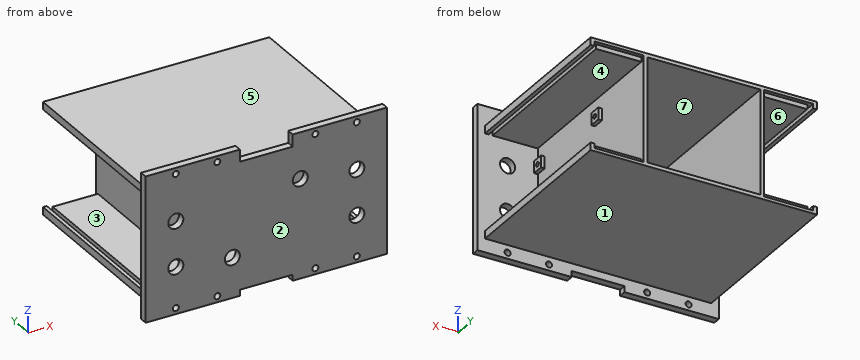
from build123d import *

# Parameters (mm, degrees)
SKETCH1_W               = 203.2
SKETCH1_H               = 203.2
BOSS_EXTRUDE1_DEPTH     = 6.35
SKETCH2_W               = 44.45
SKETCH2_H               = 45.72
SKETCH2_H_2             = 50.8
CUT_EXTRUDE1_DEPTH      = 144.824345992
SKETCH3_R               = 2.54
SKETCH3_W               = 25.4
SKETCH3_H               = 25.4
CUT_EXTRUDE2_DEPTH      = 6.35
MIRROR2_COPY_1_SKETCH_R = 2.54
MIRROR2_COPY_1_SKETCH_W = 25.4
MIRROR2_COPY_1_SKETCH_H = 25.4
MIRROR2_COPY_1_DEPTH    = 6.35
SKETCH4_W               = 101.6
SKETCH4_H               = 93.98
SKETCH4_W_2             = 95.25
SKETCH4_H_2             = 87.63
BOSS_EXTRUDE2_DEPTH     = 152.4
SKETCH5_W               = 10
SKETCH5_H               = 10
SKETCH5_R               = 1.6
BOSS_EXTRUDE3_DEPTH     = 3.175
CUT_EXTRUDE3_REACH      = 246.393
SKETCH8_R               = 1.905
SKETCH9_W               = 6.35
SKETCH9_H               = 152.4
BOSS_EXTRUDE4_DEPTH     = 44.45
SKETCH12_W              = 3.175
SKETCH12_H              = 3.81
CUT_EXTRUDE4_DEPTH      = 152.4
SKETCH13_W              = 38.1
SKETCH13_H              = 3.81
CUT_EXTRUDE5_DEPTH      = 3.175
SKETCH14_W              = 6.35
SKETCH14_H              = 152.4
BOSS_EXTRUDE5_DEPTH     = 44.45
SKETCH15_W              = 3.175
SKETCH15_H              = 3.81
CUT_EXTRUDE6_DEPTH      = 152.4
SKETCH16_W              = 38.1
SKETCH16_H              = 3.81
CUT_EXTRUDE7_DEPTH      = 3.175
CUT_EXTRUDE8_REACH      = 211.454
SKETCH17_R              = 6.35
MIRROR5_OUTLINE_R       = 6.35
MIRROR5_DEPTH           = 6.35
SKETCH18_W              = 79.375
SKETCH18_H              = 40.64
CUT_EXTRUDE9_DEPTH      = 210.453765781


# Read off the part's stored shape, not the designer's step: Mirror5
with BuildPart() as part:
    # Sketch1 → Boss-Extrude1 (new body)
    with BuildSketch(Plane(origin=(0, 0, 0), x_dir=(1, 0, 0), z_dir=(0, 1, 0))):
        Rectangle(SKETCH1_W, SKETCH1_H)
    extrude(amount=BOSS_EXTRUDE1_DEPTH)

    # Sketch2 → Cut-Extrude1 (cut, through all)
    with BuildSketch(Plane(origin=(0, 6.35, 0), x_dir=(1, 0, 0), z_dir=(0, 1, 0))):
        with Locations((0, 78.74)):
            Rectangle(SKETCH2_W, SKETCH2_H)
        with Locations((0, -76.2)):
            Rectangle(SKETCH2_W, SKETCH2_H_2)
    extrude(amount=-CUT_EXTRUDE1_DEPTH, mode=Mode.SUBTRACT)

    # Sketch3 → Cut-Extrude2 (cut)
    with BuildSketch(Plane(origin=(0, 6.35, 0), x_dir=(1, 0, 0), z_dir=(0, 1, 0))):
        with Locations(Location((-96.52, 76.2, 0), (0, 0, 270))):
            Circle(SKETCH3_R)
        with Locations(Location((-76.2, 96.52, 0), (0, 0, 270))):
            Circle(SKETCH3_R)
        with Locations(Location((-76.2, 55.88, 0), (0, 0, 270))):
            Circle(SKETCH3_R)
        with Locations(Location((-41.275, 96.52, 0), (0, 0, 270))):
            Circle(SKETCH3_R)
        with Locations(Location((-41.275, 55.88, 0), (0, 0, 90))):
            Circle(SKETCH3_R)
        with Locations((-41.148, 76.2)):
            Rectangle(SKETCH3_W, SKETCH3_H)
        with Locations((-76.2, 76.2)):
            Rectangle(SKETCH3_W, SKETCH3_H)
    cut_extrude2 = extrude(amount=-CUT_EXTRUDE2_DEPTH, mode=Mode.SUBTRACT)

    # Mirror1: Cut-Extrude2 across plane
    add(cut_extrude2.mirror(Plane(origin=(0, 0, 0), x_dir=(0, 0, 1), z_dir=(1, 0, 0))), mode=Mode.SUBTRACT)

    # Mirror2: Cut-Extrude2 across plane
    add(cut_extrude2.mirror(Plane.XY), mode=Mode.SUBTRACT)

    # Mirror2 copy 1 sketch → Mirror2 copy 1 (cut)
    with BuildSketch(Plane(origin=(0, 6.35, 0), x_dir=(-1, 0, 0), z_dir=(0, 1, 0))):
        with Locations(Location((-96.52, 76.2, 0), (0, 0, 270))):
            Circle(MIRROR2_COPY_1_SKETCH_R)
        with Locations(Location((-76.2, 96.52, 0), (0, 0, 270))):
            Circle(MIRROR2_COPY_1_SKETCH_R)
        with Locations(Location((-76.2, 55.88, 0), (0, 0, 270))):
            Circle(MIRROR2_COPY_1_SKETCH_R)
        with Locations(Location((-41.275, 96.52, 0), (0, 0, 270))):
            Circle(MIRROR2_COPY_1_SKETCH_R)
        with Locations(Location((-41.275, 55.88, 0), (0, 0, 90))):
            Circle(MIRROR2_COPY_1_SKETCH_R)
        with Locations((-41.148, 76.2)):
            Rectangle(MIRROR2_COPY_1_SKETCH_W, MIRROR2_COPY_1_SKETCH_H)
        with Locations((-76.2, 76.2)):
            Rectangle(MIRROR2_COPY_1_SKETCH_W, MIRROR2_COPY_1_SKETCH_H)
    extrude(amount=-MIRROR2_COPY_1_DEPTH, mode=Mode.SUBTRACT)

    # Sketch4 → Boss-Extrude2 (add)
    with BuildSketch(Plane(origin=(0, 6.35, 0), x_dir=(1, 0, 0), z_dir=(0, 1, 0))):
        with Locations((0, 2.54)):
            Rectangle(SKETCH4_W, SKETCH4_H)
        with Locations((0, 2.54)):
            Rectangle(SKETCH4_W_2, SKETCH4_H_2, mode=Mode.SUBTRACT)
    extrude(amount=BOSS_EXTRUDE2_DEPTH)

    # Sketch5 → Boss-Extrude3 (add)
    # profile 1 of 4: a face of its own
    with BuildSketch(Plane(origin=(50.8, 0, 0), x_dir=(0, 0, -1), z_dir=(1, 0, 0))):
        with Locations((-21.59, 93.98)):
            Rectangle(SKETCH5_W, SKETCH5_H)
        with Locations((-21.59, 93.98)):
            Circle(SKETCH5_R, mode=Mode.SUBTRACT)
    # profile 2 of 4: a face of its own
    with BuildSketch(Plane(origin=(50.8, 0, 0), x_dir=(0, 0, -1), z_dir=(1, 0, 0))):
        with Locations((26.67, 92.71)):
            Rectangle(SKETCH5_W, SKETCH5_H)
        with Locations((26.67, 92.71)):
            Circle(SKETCH5_R, mode=Mode.SUBTRACT)
    # profile 3 of 4: a face of its own
    with BuildSketch(Plane(origin=(50.8, 0, 0), x_dir=(0, 0, -1), z_dir=(1, 0, 0))):
        with Locations((-21.59, 11.43)):
            Rectangle(SKETCH5_W, SKETCH5_H)
        with Locations((-21.59, 11.43)):
            Circle(SKETCH5_R, mode=Mode.SUBTRACT)
    # profile 4 of 4: a face of its own
    with BuildSketch(Plane(origin=(50.8, 0, 0), x_dir=(0, 0, -1), z_dir=(1, 0, 0))):
        with Locations((26.67, 17.78)):
            Rectangle(SKETCH5_W, SKETCH5_H)
        with Locations((26.67, 17.78)):
            Circle(SKETCH5_R, mode=Mode.SUBTRACT)
    extrude(amount=BOSS_EXTRUDE3_DEPTH)

    # Sketch8 → Cut-Extrude3 (cut, up to next)
    with BuildSketch(Plane(origin=(53.975, 0, 0), x_dir=(0, 0, -1), z_dir=(1, 0, 0)), mode=Mode.PRIVATE) as cut_extrude3_sk1:
        with Locations((-21.59, 93.98)):
            Circle(SKETCH8_R)
    cut_extrude3_tool1 = extrude(cut_extrude3_sk1.sketch, amount=-CUT_EXTRUDE3_REACH, mode=Mode.PRIVATE) & part.part
    # Sketch8 → Cut-Extrude3 (cut, up to next)
    with BuildSketch(Plane(origin=(53.975, 0, 0), x_dir=(0, 0, -1), z_dir=(1, 0, 0)), mode=Mode.PRIVATE) as cut_extrude3_sk2:
        with Locations((26.67, 92.71)):
            Circle(SKETCH8_R)
    cut_extrude3_tool2 = extrude(cut_extrude3_sk2.sketch, amount=-CUT_EXTRUDE3_REACH, mode=Mode.PRIVATE) & part.part
    # Sketch8 → Cut-Extrude3 (cut, up to next)
    with BuildSketch(Plane(origin=(53.975, 0, 0), x_dir=(0, 0, -1), z_dir=(1, 0, 0)), mode=Mode.PRIVATE) as cut_extrude3_sk3:
        with Locations((-21.59, 11.43)):
            Circle(SKETCH8_R)
    cut_extrude3_tool3 = extrude(cut_extrude3_sk3.sketch, amount=-CUT_EXTRUDE3_REACH, mode=Mode.PRIVATE) & part.part
    # Sketch8 → Cut-Extrude3 (cut, up to next)
    with BuildSketch(Plane(origin=(53.975, 0, 0), x_dir=(0, 0, -1), z_dir=(1, 0, 0)), mode=Mode.PRIVATE) as cut_extrude3_sk4:
        with Locations((26.67, 17.78)):
            Circle(SKETCH8_R)
    cut_extrude3_tool4 = extrude(cut_extrude3_sk4.sketch, amount=-CUT_EXTRUDE3_REACH, mode=Mode.PRIVATE) & part.part
    add(cut_extrude3_tool1.solids().sort_by_distance((53.975, 93.98, 21.59))[0], mode=Mode.SUBTRACT)
    add(cut_extrude3_tool2.solids().sort_by_distance((53.975, 92.71, -26.67))[0], mode=Mode.SUBTRACT)
    add(cut_extrude3_tool3.solids().sort_by_distance((53.975, 11.43, 21.59))[0], mode=Mode.SUBTRACT)
    add(cut_extrude3_tool4.solids().sort_by_distance((53.975, 17.78, -26.67))[0], mode=Mode.SUBTRACT)

    # Sketch9 → Boss-Extrude4 (add)
    with BuildSketch(Plane(origin=(50.8, 0, 0), x_dir=(0, 0, -1), z_dir=(1, 0, 0))):
        with Locations((-41.275, 82.55)):
            Rectangle(SKETCH9_W, SKETCH9_H)
        with Locations((46.355, 82.55)):
            Rectangle(SKETCH9_W, SKETCH9_H)
    extrude(amount=BOSS_EXTRUDE4_DEPTH)

    # Sketch12 → Cut-Extrude4 (cut)
    with BuildSketch(Plane(origin=(0, 158.75, 0), x_dir=(1, 0, 0), z_dir=(0, 1, 0))):
        with Locations((90.4875, -40.005)):
            Rectangle(SKETCH12_W, SKETCH12_H)
    cut_extrude4 = extrude(amount=-CUT_EXTRUDE4_DEPTH, mode=Mode.SUBTRACT)

    # Sketch13 → Cut-Extrude5 (cut)
    with BuildSketch(Plane(origin=(0, 158.75, 0), x_dir=(1, 0, 0), z_dir=(0, 1, 0))):
        with Locations((69.85, -40.005)):
            Rectangle(SKETCH13_W, SKETCH13_H)
    cut_extrude5 = extrude(amount=-CUT_EXTRUDE5_DEPTH, mode=Mode.SUBTRACT)

    # Mirror3: Cut-Extrude4, Cut-Extrude5 across plane
    add(cut_extrude4.mirror(Plane(origin=(0, 0, -2.54), x_dir=(1, 0, 0), z_dir=(0, 0, -1))), mode=Mode.SUBTRACT)
    add(cut_extrude5.mirror(Plane(origin=(0, 0, -2.54), x_dir=(1, 0, 0), z_dir=(0, 0, -1))), mode=Mode.SUBTRACT)

    # Sketch14 → Boss-Extrude5 (add)
    with BuildSketch(Plane.ZY.offset(50.8)):
        with Locations((-46.355, 82.55)):
            Rectangle(SKETCH14_W, SKETCH14_H)
        with Locations((41.275, 82.55)):
            Rectangle(SKETCH14_W, SKETCH14_H)
    extrude(amount=BOSS_EXTRUDE5_DEPTH)

    # Sketch15 → Cut-Extrude6 (cut)
    with BuildSketch(Plane(origin=(0, 158.75, 0), x_dir=(1, 0, 0), z_dir=(0, 1, 0))):
        with Locations((-90.4875, -40.005)):
            Rectangle(SKETCH15_W, SKETCH15_H)
    cut_extrude6 = extrude(amount=-CUT_EXTRUDE6_DEPTH, mode=Mode.SUBTRACT)

    # Sketch16 → Cut-Extrude7 (cut)
    with BuildSketch(Plane(origin=(0, 158.75, 0), x_dir=(1, 0, 0), z_dir=(0, 1, 0))):
        with Locations((-69.85, -40.005)):
            Rectangle(SKETCH16_W, SKETCH16_H)
    cut_extrude7 = extrude(amount=-CUT_EXTRUDE7_DEPTH, mode=Mode.SUBTRACT)

    # Mirror4: Cut-Extrude6, Cut-Extrude7 across plane
    add(cut_extrude6.mirror(Plane(origin=(0, 0, -2.54), x_dir=(1, 0, 0), z_dir=(0, 0, -1))), mode=Mode.SUBTRACT)
    add(cut_extrude7.mirror(Plane(origin=(0, 0, -2.54), x_dir=(1, 0, 0), z_dir=(0, 0, -1))), mode=Mode.SUBTRACT)

    # Sketch17 → Cut-Extrude8 (cut, up to next)
    with BuildSketch(Plane(origin=(0, 6.35, 0), x_dir=(1, 0, 0), z_dir=(0, 1, 0)), mode=Mode.PRIVATE) as cut_extrude8_sk1:
        with Locations(Location((-76.2, -16.51, 0), (0, 0, 270))):
            Circle(SKETCH17_R)
    cut_extrude8_tool1 = extrude(cut_extrude8_sk1.sketch, amount=-CUT_EXTRUDE8_REACH, mode=Mode.PRIVATE) & part.part
    # Sketch17 → Cut-Extrude8 (cut, up to next)
    with BuildSketch(Plane(origin=(0, 6.35, 0), x_dir=(1, 0, 0), z_dir=(0, 1, 0)), mode=Mode.PRIVATE) as cut_extrude8_sk2:
        with Locations(Location((-76.2, 21.59, 0), (0, 0, 90))):
            Circle(SKETCH17_R)
    cut_extrude8_tool2 = extrude(cut_extrude8_sk2.sketch, amount=-CUT_EXTRUDE8_REACH, mode=Mode.PRIVATE) & part.part
    # Sketch17 → Cut-Extrude8 (cut, up to next)
    with BuildSketch(Plane(origin=(0, 6.35, 0), x_dir=(1, 0, 0), z_dir=(0, 1, 0)), mode=Mode.PRIVATE) as cut_extrude8_sk3:
        with Locations(Location((-28.575, 27.305, 0), (0, 0, 270))):
            Circle(SKETCH17_R)
    cut_extrude8_tool3 = extrude(cut_extrude8_sk3.sketch, amount=-CUT_EXTRUDE8_REACH, mode=Mode.PRIVATE) & part.part
    # Sketch17 → Cut-Extrude8 (cut, up to next)
    with BuildSketch(Plane(origin=(0, 6.35, 0), x_dir=(1, 0, 0), z_dir=(0, 1, 0)), mode=Mode.PRIVATE) as cut_extrude8_sk4:
        with Locations(Location((28.575, -22.225, 0), (0, 0, 270))):
            Circle(SKETCH17_R)
    cut_extrude8_tool4 = extrude(cut_extrude8_sk4.sketch, amount=-CUT_EXTRUDE8_REACH, mode=Mode.PRIVATE) & part.part
    add(cut_extrude8_tool1.solids().sort_by_distance((-76.2, 6.35, 16.51))[0], mode=Mode.SUBTRACT)
    add(cut_extrude8_tool2.solids().sort_by_distance((-76.2, 6.35, -21.59))[0], mode=Mode.SUBTRACT)
    add(cut_extrude8_tool3.solids().sort_by_distance((-28.575, 6.35, -27.305))[0], mode=Mode.SUBTRACT)
    add(cut_extrude8_tool4.solids().sort_by_distance((28.575, 6.35, 22.225))[0], mode=Mode.SUBTRACT)

    # Mirror5 outline → Mirror5 (cut)
    with BuildSketch(Plane(origin=(0, 0, 0), x_dir=(1, 0, 0), z_dir=(0, 1, 0))):
        with Locations((76.2, 21.59)):
            Circle(MIRROR5_OUTLINE_R)
        with Locations((76.2, -16.51)):
            Circle(MIRROR5_OUTLINE_R)
    extrude(amount=MIRROR5_DEPTH, mode=Mode.SUBTRACT)

    # Sketch18 → Cut-Extrude9 (cut, through all)
    with BuildSketch(Plane(origin=(0, 6.35, 0), x_dir=(1, 0, 0), z_dir=(0, 1, 0))):
        with Locations((-61.9125, 81.28)):
            Rectangle(SKETCH18_W, SKETCH18_H)
        with Locations((61.9125, 81.28)):
            Rectangle(SKETCH18_W, SKETCH18_H)
        with Locations((-61.9125, -81.28)):
            Rectangle(SKETCH18_W, SKETCH18_H)
        with Locations((61.9125, -81.28)):
            Rectangle(SKETCH18_W, SKETCH18_H)
    extrude(amount=-CUT_EXTRUDE9_DEPTH, mode=Mode.SUBTRACT)


solid = part.part
For this review, take the finished solid that the model builds, in its own axes (mm). Face numbers are marked on the shaded views. A direction names the side the tool comes from. Round coordinates to 2 decimals unless told otherwise and drop trailing zeros. Loops run counter-clockwise (first coordinate to the right, second up) from the corner with the lowest first, then second, coordinate; pieces in that order, holes last. Notation, with made-up numbers: (26.5, -33.75) - (49.5, -33.75) arc R14 ccw to (49.5, -16.75) - close; hole circle Ø3 at (82.5, -32). An arc over 180 degrees is marked (long way). One line per question, with ' | ' between items.
Q1. Take a section at C-C (z = 47.5). Give the boundary of the cut face in (x, y), and give its area (3 significant figures).
Taken from the geometry:
outline: (-101.6, 0) - (101.6, 0) - (101.6, 6.35) - (-101.6, 6.35) - close | area: 1,290 mm²
Q2. The part is to be moulded in two halves that separate along Z. For the marked faces 1, 2 and 3, say which applies: released by +Z, released by -Z, zero draft, split by the parting line, or undercut.
Taken from the geometry:
face 1: released by -Z | face 2: zero draft | face 3: undercut
Q3. For line 1 along X through (y, z) = (4.25, 55.88) (3 decimals); line 2 along Y through (x, z) = (52, -26.67) (3 decimals); line 3 along Z through (x, y) = (-76, 3), list the stretches that pass through material, from the lowest coordinate up. Write a range as [from, to].
Taken from the geometry:
line 1: x = [-101.6, -78.74], [-73.66, -43.815], [-38.735, -22.225], [22.225, 38.735], [43.815, 73.66], [78.74, 101.6] | line 2: y = [0, 6.35], [12.78, 15.875], [19.685, 22.78], [87.71, 90.805], [94.615, 97.71] | line 3: z = [-60.96, -58.41], [-53.35, -27.94], [-15.24, 10.16], [22.86, 53.35], [58.41, 60.96]
Q4. For pin 1 (12 mm diameter, centred on x = 38, y = 41, fed in from +Z); pin 2 (1.9 mm diameter, centred on y = 93, z = -46, fed in from -X); pin 3 (1 mm diameter, centred on x = -54, z = 9, fed in from +Y), all flat-tipped, find the tip position at first contact; note any pin that passes through.
Taken from the geometry:
pin 1: stops at z = 44.45 | pin 2: stops at x = -95.25 | pin 3: stops at y = 6.35
Q5. Tool access review of the marked faces 4, 5, 6 and 7: name each direction out of +Z, -Z, +X, -X, +Y, -Y from which nothing blocks a thin tool from reaching the whole face with its end or side.
Taken from the geometry:
face 4: +X, +Y | face 5: +Z, +X, -X, +Y | face 6: -X, +Y | face 7: +Y
Q6. Take a section at B-B (z = -39.5). Give the boundary of the cut face in (x, y) (3 decimals), and give its area (3 significant figures).
Taken from the geometry:
outline: (-101.6, 0) - (101.6, 0) - (101.6, 6.35) - (50.8, 6.35) - (50.8, 158.75) - (47.625, 158.75) - (47.625, 6.35) - (-47.625, 6.35) - (-47.625, 158.75) - (-50.8, 158.75) - (-50.8, 6.35) - (-101.6, 6.35) - close | area: 2,260 mm²
